Input: part model. Units: mm. Frame: model coordinates. A direction names the side the tool comes from. Round coordinates to 2 decimals unless told otherwise and drop trailing zeros. Write each loop counter-clockwise with the first axis right and the second up, starting at its lowest first coordinate (ties: lowest second). Pieces come first, ordered by that corner, then holes. Notation, with made-up numbers: M 21.25,-31 L 73.25,-31 A19 cw 73.25,-12 Z; hole C 46.25,67.25 d6. An arc over 180 degrees is marked long. Answer as CSV lines item,"result". Start each with the question number.
```python
from build123d import *

# Parameters (mm, degrees)
BOSS_EXTRUDE1_DEPTH   = 49.8
SKETCH1_R             = 8.35
BOSS_EXTRUDE1_2_DEPTH = 49.8
BOSS_EXTRUDE1_3_DEPTH = 49.8
SKETCH2_W             = 48.5
SKETCH2_H             = 16.7
BOSS_EXTRUDE2_DEPTH   = 7.2
SKETCH3_W             = 48.5
SKETCH3_H             = 16.7
BOSS_EXTRUDE3_DEPTH   = 7.2


with BuildPart() as part:
    # Sketch1 → Boss-Extrude1 (new body)
    with BuildSketch(Plane(origin=(0, 0, 0), x_dir=(1, 0, 0), z_dir=(0, 1, 0))):
        with BuildLine():
            Line((-16.002499805, 8.35), (-24.25, 8.35))
            Line((-24.25, 8.35), (-24.25, -8.35))
            Line((-24.25, -8.35), (-16.002499805, -8.35))
            ThreePointArc((-16.002499805, -8.35), (-18.05, 0), (-16.002499805, 8.35))
        make_face()
    extrude(amount=BOSS_EXTRUDE1_DEPTH)



with BuildPart() as body_2:
    # Sketch1 → Boss-Extrude1 2 (new body)
    with BuildSketch(Plane(origin=(0, 0, 0), x_dir=(1, 0, 0), z_dir=(0, 1, 0))):
        Circle(SKETCH1_R)
    extrude(amount=BOSS_EXTRUDE1_2_DEPTH)


with BuildPart() as body_3:
    # Sketch1 → Boss-Extrude1 3 (new body)
    with BuildSketch(Plane(origin=(0, 0, 0), x_dir=(1, 0, 0), z_dir=(0, 1, 0))):
        with BuildLine():
            Line((24.25, 8.35), (16.002499805, 8.35))
            ThreePointArc((16.002499805, 8.35), (17.53065346, 4.298684597), (18.05, 0))
            ThreePointArc((18.05, 0), (17.53065346, -4.298684597), (16.002499805, -8.35))
            Line((16.002499805, -8.35), (24.25, -8.35))
            Line((24.25, -8.35), (24.25, 8.35))
        make_face()
    extrude(amount=BOSS_EXTRUDE1_3_DEPTH)


with BuildPart() as part_1:
    add(part.part)

    add(body_2.part)  # Boss-Extrude2 merges body 2

    add(body_3.part)  # Boss-Extrude2 merges body 3
    # Sketch2 → Boss-Extrude2 (add)
    with BuildSketch(Plane(origin=(0, 49.8, 0), x_dir=(1, 0, 0), z_dir=(0, 1, 0))):
        Rectangle(SKETCH2_W, SKETCH2_H)
    extrude(amount=-BOSS_EXTRUDE2_DEPTH)

    # Sketch3 → Boss-Extrude3 (add)
    with BuildSketch(Plane.XZ):
        Rectangle(SKETCH3_W, SKETCH3_H)
    extrude(amount=-BOSS_EXTRUDE3_DEPTH)


solid = part_1.part
```
Item 1: Cut plane C-C, the plane z = -1.5. Return loops of the section in (x, y), plus the area to 3 significant figures.
Item 2: Access query for faces 1 (the face through (24.25, 25, 0)), 2 (the face through (13, 42.6, 0)). Directions: +Z, -Z, +X, -X, +Y, -Y. A direction counts if a zero-diameter tool reaches every point of the face in a straight line with its end or side. Return the directions, or none.
Item 3: Cut plane A-A, the plane x = 12. Return loops of the section in (y, z), plus the area to 3 significant figures.
Item 4: Draft query along Z for faces 3 (the face through (0, 49.8, 0)), 4 (the face through (-18.05, 24.65, 0.12)), 5 (the face through (17, 25, -8.35)). Return one class per face: +Z half, -Z half, draft (parallel to the pull), parting line (faces both ways), or undercut.
Item 5: Line query: line 1 (Y direction, x = 9.5, z = 0.5); line 2 (X direction, y = 40.5, z = 6); line 3 (X direction, y = 24.5, z = -7.5). Output: solid intervals per line, ascending. Write a range as [from, to].
Item 6: Cut plane B-B, the plane y = 10. Return loops of the section in (x, z).
Item 7: Cut plane D-D, the plane x = -5. Return loops of the section in (y, z), plus the area to 3 significant figures.
Results list:
1,outline,"M -24.25,0 L 24.25,0 L 24.25,49.8 L -24.25,49.8 Z; hole M -17.99,7.2 L -8.21,7.2 L -8.21,42.6 L -17.99,42.6 Z; hole M 8.21,7.2 L 17.99,7.2 L 17.99,42.6 L 8.21,42.6 Z"
1,area,"1,720 mm²"
2,face 1,"+Z, -Z, +X, +Y, -Y"
2,face 2,"none"
3,outline,"M 0,-8.35 L 7.2,-8.35 L 7.2,8.35 L 0,8.35 Z; M 42.6,-8.35 L 49.8,-8.35 L 49.8,8.35 L 42.6,8.35 Z"
3,area,"240 mm²"
4,face 3,"draft"
4,face 4,"undercut"
4,face 5,"-Z half"
5,line 1,"[0, 7.2], [42.6, 49.8]"
5,line 2,"[-24.25, -17.02], [-5.81, 5.81], [17.02, 24.25]"
5,line 3,"[-24.25, -16.42], [-3.67, 3.67], [16.42, 24.25]"
6,outline,"M -24.25,-8.35 L -16,-8.35 A18.05 cw -16,8.35 L -24.25,8.35 Z; C 0,0 d16.7; M 16,-8.35 L 24.25,-8.35 L 24.25,8.35 L 16,8.35 A18.05 cw Z"
7,outline,"M 0,-8.35 L 7.2,-8.35 L 7.2,-6.69 L 42.6,-6.69 L 42.6,-8.35 L 49.8,-8.35 L 49.8,8.35 L 42.6,8.35 L 42.6,6.69 L 7.2,6.69 L 7.2,8.35 L 0,8.35 Z"
7,area,"714 mm²"
